Build history of the part. All positions in model axes, mm. Coordinates: 2 decimals unless noted, no trailing zeros. Order: outer loops, then holes, each group sorted by start corner. A loop starts at its lowest first (then second) coordinate and runs counter-clockwise, first axis right, second up. Notation, with made-up numbers: (83.25, -38.5) -> (109.25, -38.5) arc R20 ccw to (109.25, -27.5) -> close; hole circle Ø6 at (-16, 36.25). An arc over 180 degrees is marked (long way). Write each question's results on one line, items separated by ' | '.
from build123d import *

# Parameters (mm, degrees)
BOSS_EXTRUDE1_DEPTH   = 838.2
F_8_0MM_DOWEL_HOLE1_D = 8


with BuildPart() as part:
    # Sketch1 → Boss-Extrude1 (new body)
    with BuildSketch(Plane.XY):
        Polygon((0, -5.318754457), (0, -13.318754457), (2.54, -13.318754457), (2.54, -18.398754457), (-5.08, -18.398754457), (-5.08, -0.238754457), (2.54, -0.238754457), (2.54, -5.318754457), align=None)
    extrude(amount=BOSS_EXTRUDE1_DEPTH)

    # Ø8.0mm Dowel Hole1 (through all)
    with Locations(Plane.ZY.offset(5.08)):
        with Locations((812.8, -9.318754457), (28.049203363, -40.337204001)):
            Hole(F_8_0MM_DOWEL_HOLE1_D / 2)


solid = part.part
Item 1: Slice it at A-A, the plane x = 1.25. List the corners of the cut face in (y, z), and give its area (3 significant figures).
Answer:
outline: (-18.4, 0) -> (-13.32, 0) -> (-13.32, 838.2) -> (-18.4, 838.2) -> close; (-5.32, 0) -> (-0.24, 0) -> (-0.24, 838.2) -> (-5.32, 838.2) -> close | area: 8,520 mm^2
Item 2: Pin check, flat tips, straight feed: pin 1 (7 mm diameter, centred on y = -9.32, z = 812.8, fed in from -X) (3 decimals); pin 2 (6.5 mm diameter, centred on y = -11, z = 829.5, fed in from +X). Stop position of each tip, or through.
Answer:
pin 1: passes through | pin 2: stops at x = 2.54
Item 3: Drill centre lines: line 1 (Y direction, x = -1.55, z = 812.8); line 2 (X direction, y = -9, z = 254); line 3 (Z direction, x = -3.5, y = -12). Where is each one in solid material? Low to high. Write a range as from..to.
Answer:
line 1: y = -18.4..-13.32, -5.32..-0.24 | line 2: x = -5.08..0 | line 3: z = 0..809.83, 815.77..838.2
Item 4: Slice it at B-B, the plane z = 616. List the corners of the cut face in (x, y).
Answer:
outline: (-5.08, -18.4) -> (2.54, -18.4) -> (2.54, -13.32) -> (0, -13.32) -> (0, -5.32) -> (2.54, -5.32) -> (2.54, -0.24) -> (-5.08, -0.24) -> close
